For this review, take the finished solid that the model builds, in its own axes (mm). Face numbers are marked on the shaded views. A direction names the side the tool comes from. Coordinates: 2 decimals unless noted, no trailing zeros. Loops run counter-clockwise (first coordinate to the right, second up) from the corner with the lowest first, then second, coordinate; pieces in that order, holes last.
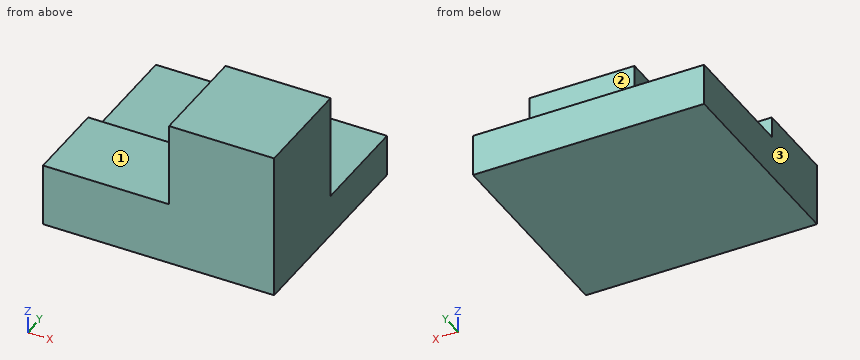
```python
from build123d import *

# Parameters (mm, degrees)
F1_DEPTH = 88.9
F0_W     = 76.2
F0_H     = 50.8
F2_DEPTH = 38.1
F3_DEPTH = 25.4


with BuildPart() as f1:
    # F0 (on Top) → F1 (new body)
    with BuildSketch(Plane.XY):
        Polygon((0, -63.5), (63.5, -63.5), (63.5, 0), (0, 0), (0, -12.7), align=None)
    extrude(amount=F1_DEPTH)

    # F0 (on Top) → F2 (join)
    with BuildSketch(Plane.XY):
        with Locations((-38.1, -38.1)):
            Rectangle(F0_W, F0_H)
    extrude(amount=F2_DEPTH)

    # F0 (on Top) → F3 (join)
    with BuildSketch(Plane.XY):
        Polygon((0, 0), (63.5, 0), (63.5, 63.5), (-76.2, 63.5), (-76.2, -12.7), (0, -12.7), align=None)
    extrude(amount=F3_DEPTH)


solid = f1.part
```
Q1. Machinability: for the marked faces 1, 2 and 3, which of the approach directions +Z, -Z, +X, -X, +Y, -Y give a long, thin tool a straight path to every point of the face, cutting with its end or side? Answer none if there is none.
Q2. Wall thickness on probe 1 along Z at (x, y) = (-63, -1.5); probe 2 along Z at (x, y) = (-6, -53.5); probe 3 along X at (y, z) = (-54, 64): over which ranges is each line inside the solid? List them lowest first.
Q3. Consider section D-D (y = 55.5). State the section outline as (x, z) points, then the cut area to 3 significant figures.
Q4. For pin 1 Ø10 at (x, y) = (-45, 11) entering from +Z; pin 2 Ø4 at (x, z) = (22, 37) entering from +Y; pin 3 Ø4 at (x, z) = (-31, 29.5) entering from +Y, all flat-tipped, find the tip position at first contact; note any pin that passes through.
Q5. Consider section C-C (z = 47.5). State the section outline as (x, y) points, then the cut area to 3 significant figures.
Q6. Consider section A-A (x = 34). State the section outline as (y, z) points, then the cut area to 3 significant figures.
Q7. Consider section B-B (y = -28). State the section outline as (x, z) points, then the cut area to 3 significant figures.
Model answer:
1. face 1: +Z, -X, +Y, -Y
1. face 2: +Z, +X, -X, +Y
1. face 3: +Z, -Z, -X, +Y, -Y
2. probe 1: z = 0 to 25.4
2. probe 2: z = 0 to 38.1
2. probe 3: x = 0 to 63.5
3. outline: (-76.2, 0) - (63.5, 0) - (63.5, 25.4) - (-76.2, 25.4) - close
3. area: 3,550 mm2
4. pin 1: stops at z = 25.4
4. pin 2: stops at y = 0
4. pin 3: stops at y = -12.7
5. outline: (0, -63.5) - (63.5, -63.5) - (63.5, 0) - (0, 0) - close
5. area: 4,030 mm2
6. outline: (-63.5, 0) - (63.5, 0) - (63.5, 25.4) - (0, 25.4) - (0, 88.9) - (-63.5, 88.9) - close
6. area: 7,260 mm2
7. outline: (-76.2, 0) - (63.5, 0) - (63.5, 88.9) - (0, 88.9) - (0, 38.1) - (-76.2, 38.1) - close
7. area: 8,550 mm2
